```python
from build123d import *

# Parameters (mm, degrees)
F0_W     = 104.5
F0_H     = 28.3
F0_W_2   = 101.5
F0_H_2   = 25.3
F1_DEPTH = 130
F2_R     = 0.875
F3_DEPTH = 130
F4_W     = 104.5
F4_H     = 28.3
F5_DEPTH = 1.5
F6_R     = 3.847092
F7_DEPTH = 3


with BuildPart() as f1:
    # F0 (on Top) → F1 (new body)
    with BuildSketch(Plane.XY):
        with Locations((-2.827974, -2.56671)):
            Rectangle(F0_W, F0_H)
        with Locations((-2.827974, -2.56671)):
            Rectangle(F0_W_2, F0_H_2, mode=Mode.SUBTRACT)
    extrude(amount=F1_DEPTH)

    # F2 (on face) → F3 (cut)
    with BuildSketch(Plane.YZ.offset(49.422026)):
        with Locations((5.58329, 114)):
            Circle(F2_R)
        with Locations((5.58329, 84)):
            Circle(F2_R)
        with Locations((5.58329, 24.5)):
            Circle(F2_R)
    extrude(amount=-F3_DEPTH, mode=Mode.SUBTRACT)

    # F4 (on face) → F5 (join)
    with BuildSketch(Plane.XY.offset(130)):
        with Locations((-2.827974, -2.56671)):
            Rectangle(F4_W, F4_H)
    extrude(amount=F5_DEPTH)

    # F6 (on face) → F7 (cut)
    with BuildSketch(Plane(origin=(0, 0, 130), x_dir=(1, 0, 0), z_dir=(0, 0, -1))):
        with Locations((-2.827974, 2.56671)):
            Circle(F6_R)
    extrude(amount=-F7_DEPTH, mode=Mode.SUBTRACT)


solid = f1.part
```
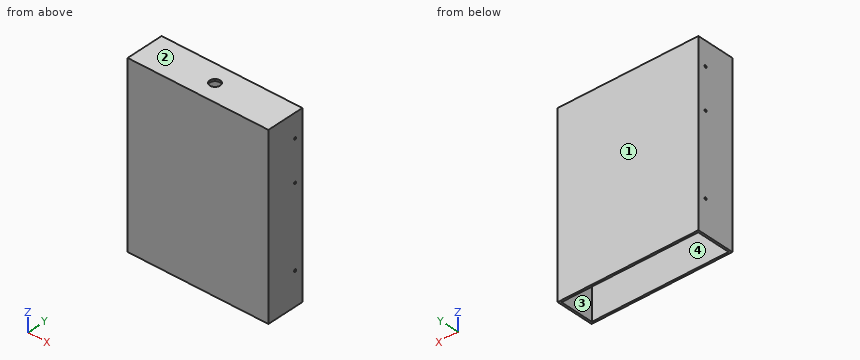
Geometry: final body of the model. Coordinates: model frame, mm. Face numbers are marked on the shaded views. Coordinates: 2 decimals unless noted, no trailing zeros. Order: outer loops, then holes, each group sorted by start corner. A loop starts at its lowest first (then second) coordinate and runs counter-clockwise, first axis right, second up. Notation, with made-up numbers: (10, 59) -> (57, 59) arc R34 ccw to (57, 90) -> close; hole circle Ø7 at (19, -29.75). An arc over 180 degrees is marked (long way). Answer in a Markdown table with one row per item.
Item 1: Section B-B on y = -8.25. Output: boundary loops of the cut face in (x, z), plus the area to 3 significant figures.
Return value:
| item | result |
|---|---|
| outline | (-55.08, 0) -> (-53.58, 0) -> (-53.58, 130) -> (47.92, 130) -> (47.92, 0) -> (49.42, 0) -> (49.42, 131.5) -> (-55.08, 131.5) -> close |
| area | 547 mm² |
Item 2: Ray query, L1, parallel to X at y = 8.75, z = 44.5; L2, parallel to Y at x = -42.5, z = 11; L3, parallel to Z at x = 18.5, y = 1. Return the intervals inside material, ascending.
Return value:
| item | result |
|---|---|
| L1 | x = -55.08 to -53.58, 47.92 to 49.42 |
| L2 | y = -16.72 to -15.22, 10.08 to 11.58 |
| L3 | z = 130 to 131.5 |
Item 3: Section C-C on x = -28. Output: boundary loops of the cut face in (y, z), plus the area to 3 significant figures.
Return value:
| item | result |
|---|---|
| outline | (-16.72, 0) -> (-15.22, 0) -> (-15.22, 130) -> (10.08, 130) -> (10.08, 0) -> (11.58, 0) -> (11.58, 131.5) -> (-16.72, 131.5) -> close |
| area | 432 mm² |
Item 4: Draft query along Y for the marked faces 1, 2, 3 and 4. Return one class per face: released by +Y, released by -Y, zero draft, split by the parting line, or undercut.
Return value:
| item | result |
|---|---|
| face 1 | released by +Y |
| face 2 | zero draft |
| face 3 | undercut |
| face 4 | undercut |
Item 5: Contact query for a flat-ended pin moving along its axis: P1, Ø2.5, axis at y = 5.58, z = 114, coming from the +X side. Output: stop coordinate, or through.
Return value:
| item | result |
|---|---|
| P1 | stops at x = 49.42 |
Item 6: Section A-A on z = 81.5. Output: boundary loops of the cut face in (x, y).
Return value:
| item | result |
|---|---|
| outline | (-55.08, -16.72) -> (49.42, -16.72) -> (49.42, 11.58) -> (-55.08, 11.58) -> close; hole (-53.58, -15.22) -> (47.92, -15.22) -> (47.92, 10.08) -> (-53.58, 10.08) -> close |
